Design review of the part shown in the three views and the two pictorial views. Dimensions are in mm from the part's minimum x, y and z. A direction names the side the tool comes from. Round coordinates to 2 decimals unless told otherwise and drop trailing zeros. Order: outer loops, then holes, each group sorted by start corner. A loop starts at its lowest first (then second) coordinate and runs counter-clockwise, first axis right, second up. Notation, with made-up numbers: (38.5, -4) - (86.5, -4) arc R24 cw to (86.5, 17) - close; hole circle Ø3 at (21, -18.75). An arc over 180 degrees is marked (long way). Use CSV: the item, a comma, the result in double quotes.
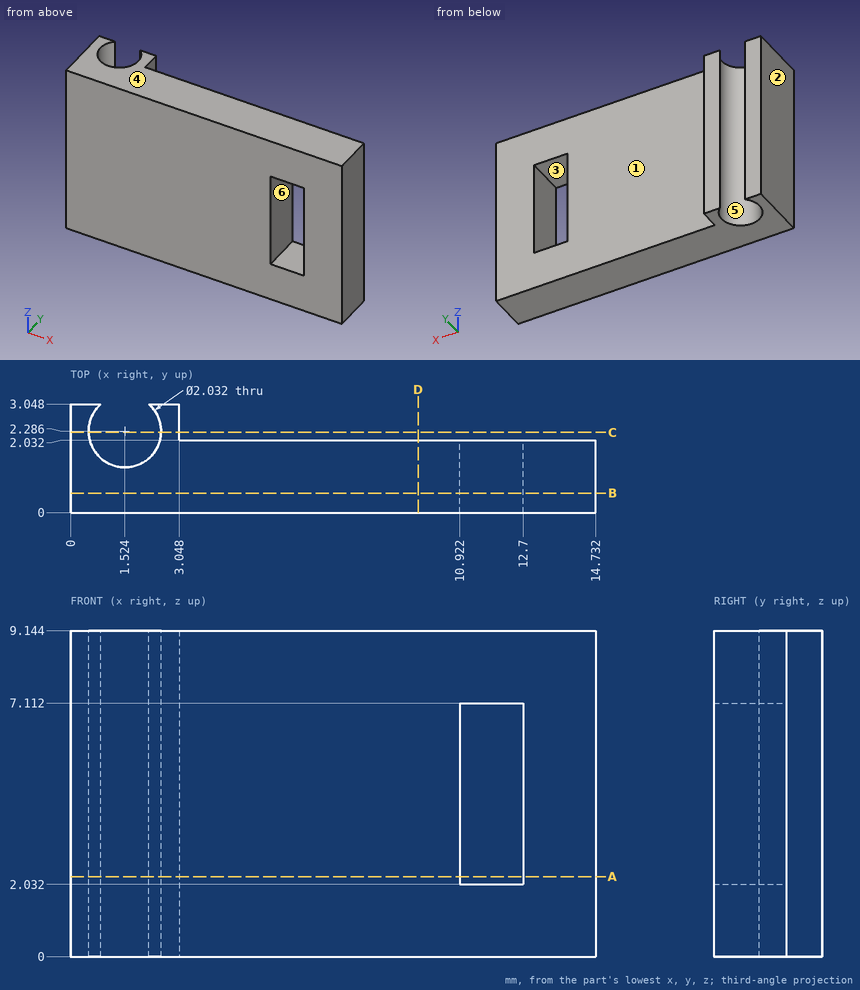
1) Insertion check: pin 1 Ø2 at (x, z) = (4.5, 7) entering from +Y. The pin has a flat end and moves straight along its axis. Give the tip position at first contact, or say it passes through.
Data:
pin 1,"stops at y = 2.03"
2) For the marked faces 1, 2 and 3, list the 3-axis set-ups (+Z, -Z, +X, -X, +Y, -Y) from which the entire face can be reached by the end or side of a thin tool; tool diameter is ignored.
Data:
face 1,"+Z, -Z, +X, +Y"
face 2,"+Z, -Z, -X, +Y, -Y"
face 3,"+Y, -Y"
3) The part is to be moulded in two halves that separate along Z. For the marked faces 4, 5 and 6, say which applies: +Z half, -Z half, draft (parallel to the pull), parting line (faces both ways), or undercut.
Data:
face 4,"+Z half"
face 5,"draft"
face 6,"undercut"
4) We need section C-C (y = 2.25). Give the boundary of the cut face in (x, z).
Data:
outline,"(0, 0) - (0.51, 0) - (0.51, 9.14) - (0, 9.14) - close; (2.54, 0) - (3.05, 0) - (3.05, 9.14) - (2.54, 9.14) - close"
5) We need section A-A (z = 2.25). Give the boundary of the cut face in (x, y), then the cut area to 3 significant figures.
Data:
outline,"(0, 0) - (10.92, 0) - (10.92, 2.03) - (3.05, 2.03) - (3.05, 3.05) - (2.2, 3.05) arc R1.02 cw (long way) to (0.85, 3.05) - (0, 3.05) - close; (12.7, 0) - (14.73, 0) - (14.73, 2.03) - (12.7, 2.03) - close"
area,"26.4 mm2"
6) We need section D-D (x = 9.75). Give the boundary of the cut face in (y, z), then the cut area to 3 significant figures.
Data:
outline,"(0, 0) - (2.03, 0) - (2.03, 9.14) - (0, 9.14) - close"
area,"18.6 mm2"
7) To check wall thickness, follow L1, parallel to Z at x = 12.5, y = 0.3; L2, parallel to Y at x = 11.75, z = 0.5; L3, parallel to X at y = 1.8, z = 6.5. State the ranges of each line that lie inside material, in increasing order. Write a range as from..to.
Data:
L1,"z = 0..2.03, 7.11..9.14"
L2,"y = 0..2.03"
L3,"x = 0..0.63, 2.42..10.92, 12.7..14.73"
8) We need section B-B (y = 0.55). Give the boundary of the cut face in (x, z).
Data:
outline,"(0, 0) - (14.73, 0) - (14.73, 9.14) - (0, 9.14) - close; hole (10.92, 2.03) - (12.7, 2.03) - (12.7, 7.11) - (10.92, 7.11) - close"
